from build123d import *

# Parameters (mm, degrees)
SKETCH1_W               = 39.032335112
SKETCH1_H               = 81.259338173
SKETCH1_R               = 3.175
BOSS_EXTRUDE1_DEPTH     = 3.175
F_1_4_28_TAPPED_HOLE1_D = 5.4102


with BuildPart() as part:
    # Sketch1 → Boss-Extrude1 (new body)
    with BuildSketch(Plane.XY):
        with Locations((-69.293997496, 206.742821462)):
            Rectangle(SKETCH1_W, SKETCH1_H)
        with Locations((-76.2, 235.857142857)):
            Circle(SKETCH1_R, mode=Mode.SUBTRACT)
        with Locations((-76.2, 176.892857143)):
            Circle(SKETCH1_R, mode=Mode.SUBTRACT)
    extrude(amount=BOSS_EXTRUDE1_DEPTH)

    # 1/4-28 Tapped Hole1 (through all)
    with Locations(Plane.XY.offset(3.175)):
        with Locations((-63.5, 205.74)):
            Hole(F_1_4_28_TAPPED_HOLE1_D / 2)


solid = part.part
Verification items for the finished model (mm, model axes). Coordinates: 2 decimals unless noted, no trailing zeros. Order: outer loops, then holes, each group sorted by start corner. A loop starts at its lowest first (then second) coordinate and runs counter-clockwise, first axis right, second up.
Item 1: Section check B-B, the plane y = 205.74. Enter the section's corners in (x, z) (3 decimals), then the cut area to 3 significant figures.
Filled in:
outline: (-88.81, 0) - (-66.205, 0) - (-66.205, 3.175) - (-88.81, 3.175) - close; (-60.795, 0) - (-49.778, 0) - (-49.778, 3.175) - (-60.795, 3.175) - close
area: 107 mm2
Item 2: Section check C-C, the plane x = -76.2. Enter the section's corners in (y, z) (1 decimal).
Filled in:
outline: (166.1, 0) - (173.7, 0) - (173.7, 3.2) - (166.1, 3.2) - close; (180.1, 0) - (232.7, 0) - (232.7, 3.2) - (180.1, 3.2) - close; (239, 0) - (247.4, 0) - (247.4, 3.2) - (239, 3.2) - close
Item 3: Release check for a two-part mould opening along Y. For faces 1 (the face through (-64.954, 208.021, 1.565)), 2 (the face through (-88.81, 206, 2)), 3 (the face through (-70, 247.372, 2)), 4 (the face through (-74.73, 174.08, 1.57)) record: +Y half, -Y half, draft (parallel to the pull), parting line (faces both ways), or undercut.
Filled in:
face 1: undercut
face 2: draft
face 3: +Y half
face 4: undercut
Item 4: Material ranges on L1, parallel to Y at x = -76.2, z = 2.35; L2, parallel to Y at x = -63.5, z = 1.55; L3, parallel to X at y = 206.5, z = 1.8, recorded low to high.
Filled in:
L1: y = 166.11 to 173.72, 180.07 to 232.68, 239.03 to 247.37
L2: y = 166.11 to 203.03, 208.45 to 247.37
L3: x = -88.81 to -66.1, -60.9 to -49.78
Item 5: Section check A-A, the plane x = -63.5. Enter the section's corners in (y, z) (1 decimal).
Filled in:
outline: (166.1, 0) - (203, 0) - (203, 3.2) - (166.1, 3.2) - close; (208.4, 0) - (247.4, 0) - (247.4, 3.2) - (208.4, 3.2) - close
Item 6: Section check D-D, the plane z = 1.85. Give the number of separate pieces and of enclosed holes in the cut face, then the cut area to 3 significant figures.
Filled in:
separate pieces: 1
enclosed holes: 3
area: 3,090 mm2
